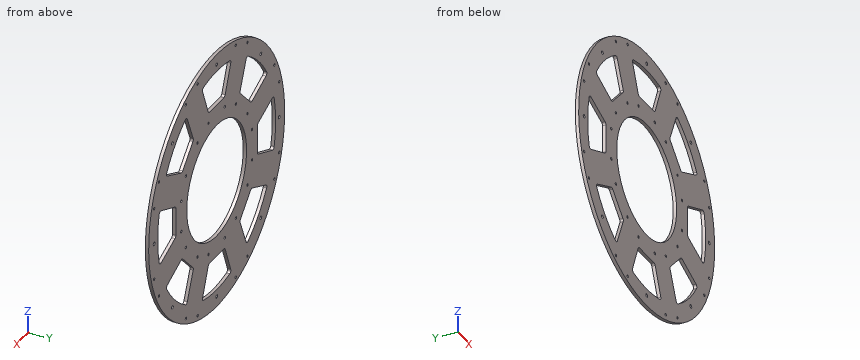
from build123d import *

# Parameters (mm, degrees)
SKETCH1_R                   = 250
SKETCH1_R_2                 = 110
BOSS_EXTRUDE1_DEPTH         = 6.35
M6_CLEARANCE_HOLE1_D        = 6.4
TAP_DRILL_FOR_M6X1_0_TAP2_D = 5
CIRPATTERN1_COUNT           = 8


with BuildPart() as part:
    # Sketch1 → Boss-Extrude1 (new body)
    with BuildSketch(Plane(origin=(0, 0, 0), x_dir=(1, 0, 0), z_dir=(0, 1, 0))):
        with Locations(Location((0, 0, 0), (0, 0, 270))):
            Circle(SKETCH1_R)
        with Locations(Location((0, 0, 0), (0, 0, 270))):
            Circle(SKETCH1_R_2, mode=Mode.SUBTRACT)
        with BuildLine():
            Line((-26.614835193, 150), (26.614835193, 150))
            ThreePointArc((26.614835193, 150), (29.417979239, 150.859663848), (31.257218647, 153.143046618))
            Line((31.257218647, 153.143046618), (51.858276397, 204.645690993))
            ThreePointArc((51.858276397, 204.645690993), (51.644491556, 208.823746337), (48.330359895, 211.376858507))
            ThreePointArc((48.330359895, 211.376858507), (0, 216.831731995), (-48.330359895, 211.376858507))
            ThreePointArc((-48.330359895, 211.376858507), (-51.644491556, 208.823746337), (-51.858276397, 204.645690993))
            Line((-51.858276397, 204.645690993), (-31.257218647, 153.143046618))
            ThreePointArc((-31.257218647, 153.143046618), (-29.417979239, 150.859663848), (-26.614835193, 150))
        make_face(mode=Mode.SUBTRACT)
        with BuildLine():
            Line((86.186295489, 130.390678022), (108.037016941, 181.375694743))
            ThreePointArc((108.037016941, 181.375694743), (111.142516918, 184.178857298), (115.291284818, 183.640735255))
            ThreePointArc((115.291284818, 183.640735255), (153.32318807, 153.32318807), (183.640735255, 115.291284818))
            ThreePointArc((183.640735255, 115.291284818), (184.178857298, 111.142516918), (181.375694743, 108.037016941))
            Line((181.375694743, 108.037016941), (130.390678022, 86.186295489))
            ThreePointArc((130.390678022, 86.186295489), (127.475543923, 85.872238705), (124.885547623, 87.246486733))
            Line((124.885547623, 87.246486733), (87.246486733, 124.885547623))
            ThreePointArc((87.246486733, 124.885547623), (85.872238705, 127.475543923), (86.186295489, 130.390678022))
        make_face(mode=Mode.SUBTRACT)
        with BuildLine():
            Line((153.143046618, 31.257218647), (204.645690993, 51.858276397))
            ThreePointArc((204.645690993, 51.858276397), (208.823746337, 51.644491556), (211.376858507, 48.330359895))
            ThreePointArc((211.376858507, 48.330359895), (216.831731995, 0), (211.376858507, -48.330359895))
            ThreePointArc((211.376858507, -48.330359895), (208.823746337, -51.644491556), (204.645690993, -51.858276397))
            Line((204.645690993, -51.858276397), (153.143046618, -31.257218647))
            ThreePointArc((153.143046618, -31.257218647), (150.859663848, -29.417979239), (150, -26.614835193))
            Line((150, -26.614835193), (150, 26.614835193))
            ThreePointArc((150, 26.614835193), (150.859663848, 29.417979239), (153.143046618, 31.257218647))
        make_face(mode=Mode.SUBTRACT)
        with BuildLine():
            Line((130.390678022, -86.186295489), (181.375694743, -108.037016941))
            ThreePointArc((181.375694743, -108.037016941), (184.178857298, -111.142516918), (183.640735255, -115.291284818))
            ThreePointArc((183.640735255, -115.291284818), (153.32318807, -153.32318807), (115.291284818, -183.640735255))
            ThreePointArc((115.291284818, -183.640735255), (111.142516918, -184.178857298), (108.037016941, -181.375694743))
            Line((108.037016941, -181.375694743), (86.186295489, -130.390678022))
            ThreePointArc((86.186295489, -130.390678022), (85.872238705, -127.475543923), (87.246486733, -124.885547623))
            Line((87.246486733, -124.885547623), (124.885547623, -87.246486733))
            ThreePointArc((124.885547623, -87.246486733), (127.475543923, -85.872238705), (130.390678022, -86.186295489))
        make_face(mode=Mode.SUBTRACT)
        with BuildLine():
            Line((31.257218647, -153.143046618), (51.858276397, -204.645690993))
            ThreePointArc((51.858276397, -204.645690993), (51.644491556, -208.823746337), (48.330359895, -211.376858507))
            ThreePointArc((48.330359895, -211.376858507), (0, -216.831731995), (-48.330359895, -211.376858507))
            ThreePointArc((-48.330359895, -211.376858507), (-51.644491556, -208.823746337), (-51.858276397, -204.645690993))
            Line((-51.858276397, -204.645690993), (-31.257218647, -153.143046618))
            ThreePointArc((-31.257218647, -153.143046618), (-29.417979239, -150.859663848), (-26.614835193, -150))
            Line((-26.614835193, -150), (26.614835193, -150))
            ThreePointArc((26.614835193, -150), (29.417979239, -150.859663848), (31.257218647, -153.143046618))
        make_face(mode=Mode.SUBTRACT)
        with BuildLine():
            Line((-86.186295489, -130.390678022), (-108.037016941, -181.375694743))
            ThreePointArc((-108.037016941, -181.375694743), (-111.142516918, -184.178857298), (-115.291284818, -183.640735255))
            ThreePointArc((-115.291284818, -183.640735255), (-153.32318807, -153.32318807), (-183.640735255, -115.291284818))
            ThreePointArc((-183.640735255, -115.291284818), (-184.178857298, -111.142516918), (-181.375694743, -108.037016941))
            Line((-181.375694743, -108.037016941), (-130.390678022, -86.186295489))
            ThreePointArc((-130.390678022, -86.186295489), (-127.475543923, -85.872238705), (-124.885547623, -87.246486733))
            Line((-124.885547623, -87.246486733), (-87.246486733, -124.885547623))
            ThreePointArc((-87.246486733, -124.885547623), (-85.872238705, -127.475543923), (-86.186295489, -130.390678022))
        make_face(mode=Mode.SUBTRACT)
        with BuildLine():
            Line((-153.143046618, -31.257218647), (-204.645690993, -51.858276397))
            ThreePointArc((-204.645690993, -51.858276397), (-208.823746337, -51.644491556), (-211.376858507, -48.330359895))
            ThreePointArc((-211.376858507, -48.330359895), (-216.831731995, 0), (-211.376858507, 48.330359895))
            ThreePointArc((-211.376858507, 48.330359895), (-208.823746337, 51.644491556), (-204.645690993, 51.858276397))
            Line((-204.645690993, 51.858276397), (-153.143046618, 31.257218647))
            ThreePointArc((-153.143046618, 31.257218647), (-150.859663848, 29.417979239), (-150, 26.614835193))
            Line((-150, 26.614835193), (-150, -26.614835193))
            ThreePointArc((-150, -26.614835193), (-150.859663848, -29.417979239), (-153.143046618, -31.257218647))
        make_face(mode=Mode.SUBTRACT)
        with BuildLine():
            Line((-130.390678022, 86.186295489), (-181.375694743, 108.037016941))
            ThreePointArc((-181.375694743, 108.037016941), (-184.178857298, 111.142516918), (-183.640735255, 115.291284818))
            ThreePointArc((-183.640735255, 115.291284818), (-153.32318807, 153.32318807), (-115.291284818, 183.640735255))
            ThreePointArc((-115.291284818, 183.640735255), (-111.142516918, 184.178857298), (-108.037016941, 181.375694743))
            Line((-108.037016941, 181.375694743), (-86.186295489, 130.390678022))
            ThreePointArc((-86.186295489, 130.390678022), (-85.872238705, 127.475543923), (-87.246486733, 124.885547623))
            Line((-87.246486733, 124.885547623), (-124.885547623, 87.246486733))
            ThreePointArc((-124.885547623, 87.246486733), (-127.475543923, 85.872238705), (-130.390678022, 86.186295489))
        make_face(mode=Mode.SUBTRACT)
    extrude(amount=-BOSS_EXTRUDE1_DEPTH)

    # M6 Clearance Hole1 (through all)
    with Locations(Plane(origin=(0, 0, -230), x_dir=(0, 0, 1), z_dir=(0, 1, 0))):
        with Locations((0, 0), (67.365440327, -162.634559673), (230, -230), (67.365440327, 162.634559673), (230, 230), (392.634559673, 162.634559673), (460, 0), (392.634559673, -162.634559673)):
            Hole(M6_CLEARANCE_HOLE1_D / 2)

    # Tap Drill for M6x1.0 Tap2 (through all)
    with Locations(Plane(origin=(-70, 0, -230), x_dir=(0, 0, 1), z_dir=(0, 1, 0))):
        with Locations((0, 0), (0, 140), (100, 100), (100, 40)):
            tap_drill_for_m6x1_0_tap2 = Hole(TAP_DRILL_FOR_M6X1_0_TAP2_D / 2)

    # CirPattern1: Tap Drill for M6x1.0 Tap2 ×8 about axis
    cirpattern1_axis = Axis((0, 0, 0), (0, 1, 0))
    for i in range(1, CIRPATTERN1_COUNT):
        add(tap_drill_for_m6x1_0_tap2.rotate(cirpattern1_axis, i * 360 / CIRPATTERN1_COUNT), mode=Mode.SUBTRACT)


solid = part.part
Geometry check sheet. Reference: the model listing, model coordinates, mm. Give positions to 0.01 mm unless a question says otherwise; leave off trailing zeros. Loops run counter-clockwise (first coordinate to the right, second up) from the corner with the lowest first, then second, coordinate; pieces in that order, holes last. Notation, with made-up numbers: M -10.75,81.25 L 32.25,81.25 A32 ccw 32.25,118.25 Z; hole C 67.25,43 d4. An arc over 180 degrees is marked long. Answer as a JSON object with one key per item and string values. Group by question number.
Item 1: Sectioned sample at B-B on x = 100.5. Record the boundary of the cut face in (y, z).
Item 2: Sectioned sample at C-C on y = -5. Give the number of separate pieces and of enclosed holes in the cut face, plus the area to 3 significant figures.
Item 3: Material ranges on L1, parallel to Z at x = 24, y = -1.5; L2, parallel to X at y = -0.75, z = 119.5; L3, parallel to Z at x = -140.5, y = -0.5, recorded low to high.
Item 4: Sectioned sample at A-A on x = 14. Record the boundary of the cut face in (y, z).
Item 5: Gauge pin test, flat ends, axial feed: pin 1 (6.5 mm diameter, centred on x = 30, z = -130, fed in from -Y); pin 2 (3 mm diameter, centred on x = 149.5, y = -5.5, fed in from +Z); pin 3 (3 mm diameter, centred on x = -96, y = -5.5, fed in from +Z); pin 4 (1 mm diameter, centred on x = -159, y = -1, fed in from +Z). Record the tip position at first contact, or that the pin passes through.
Findings below:
{
 "1": {"outline": "M -6.35,-228.91 L 0,-228.91 L 0,-163.79 L -6.35,-163.79 Z; M -6.35,-111.63 L 0,-111.63 L 0,-44.72 L -6.35,-44.72 Z; M -6.35,44.72 L 0,44.72 L 0,111.63 L -6.35,111.63 Z; M -6.35,163.79 L 0,163.79 L 0,228.91 L -6.35,228.91 Z"},
 "2": {"separate pieces": "1", "enclosed holes": "49", "area": "113,000 mm2"},
 "3": {"L1": "-248.85 to -215.5, -150 to -107.35, 107.35 to 150, 215.5 to 248.85", "L2": "-219.59 to -180.93, -92.63 to 92.63, 180.93 to 219.59", "L3": "-206.78 to -165.15, -90.52 to 90.52, 165.15 to 206.78"},
 "4": {"outline": "M -6.35,-249.61 L 0,-249.61 L 0,-216.38 L -6.35,-216.38 Z; M -6.35,-150 L 0,-150 L 0,-109.11 L -6.35,-109.11 Z; M -6.35,109.11 L 0,109.11 L 0,150 L -6.35,150 Z; M -6.35,216.38 L 0,216.38 L 0,249.61 L -6.35,249.61 Z"},
 "5": {"pin 1": "y = -6.35", "pin 2": "z = 201.48", "pin 3": "z = 231.45", "pin 4": "z = 193.33"}
}
